Here's how the part is built. I have some questions about the finished solid (model axes, mm). A direction names the side the tool comes from. Coordinates: 2 decimals unless noted, no trailing zeros. Write each loop counter-clockwise with the first axis right and the second up, starting at its lowest first coordinate (ties: lowest second). Pieces come first, ordered by that corner, then holes.
```python
from build123d import *

# Parameters (mm, degrees)
F1_DEPTH = 903
F4_DEPTH = 5
F5_R     = 2


# Not quite as in the source:
# - a feature names something its author has since deleted; it is built from what else it names


with BuildPart() as f1:
    # F0 (on Right) → F1 (new body)
    with BuildSketch(Plane.YZ):
        Polygon((-295, 0), (0, 0), (0, 430), (-5, 430), (-5, 5), (-290, 5), (-290, 430), (-295, 430), align=None)
    extrude(amount=F1_DEPTH)

    # F3 (on offset) → F4 (join)
    with BuildSketch(Plane.YZ.offset(300)):
        Polygon((-230, 0), (-5, 0), (-5, 360), align=None)
    extrude(amount=F4_DEPTH)

    # F5
    f5_edges = [f1.edges().sort_by_distance(p)[0] for p in [
        (451.5, 0, 0),
        (451.5, -295, 0),
    ]]
    fillet(f5_edges, radius=F5_R)


solid = f1.part
```
1) Will these pins go through, and if not, where does the flat tip stop? pin 1 (5 mm diameter, centred on y = -156, z = 87.5, fed in from +X); pin 2 (6 mm diameter, centred on x = 108.5, y = -62.5, fed in from +Z).
Values follow:
pin 1: stops at x = 305
pin 2: stops at z = 5
2) Imagine slicing it at B-B on z = 327.5. Please give me the cut outline in (x, y).
Values follow:
outline: (0, -295) - (903, -295) - (903, -290) - (0, -290) - close; (0, -5) - (300, -5) - (300, -25.31) - (305, -25.31) - (305, -5) - (903, -5) - (903, 0) - (0, 0) - close
3) Imagine slicing it at A-A on y = -189. Please give me the cut outline in (x, z).
Values follow:
outline: (0, 0) - (903, 0) - (903, 5) - (305, 5) - (305, 65.6) - (300, 65.6) - (300, 5) - (0, 5) - close
4) On a 3-axis mill with a long thin cutter (end or side, diameter ignored), from which of +Z, -Z, +X, -X, +Y, -Y can I reach the whole of each face in a straight line? I mean faces 4 (the face through (302.465, -114.384, 184.985)), 5 (the face through (445, -295, 219)), 6 (the face through (445, -5, 220)), 7 (the face through (305, -68, 106)). Say none if no direction works.
Values follow:
face 4: +Z, +X, -X
face 5: +Z, -Z, +X, -X, -Y
face 6: +Z
face 7: +Z, +X
5) I need wall thicknesses on probe 1 along Y at (x, z) = (498, 99.5); probe 2 along Z at (x, y) = (800, -122.5); probe 3 along X at (y, z) = (-76.5, 118). Which ranges of each line are inside material? Lowest first, please.
Values follow:
probe 1: y = -295 to -290, -5 to 0
probe 2: z = 0 to 5
probe 3: x = 300 to 305
6) Imagine slicing it at C-C on x = 614. Please give me the cut outline in (y, z).
Values follow:
outline: (-295, 2) arc R2 ccw to (-293, 0) - (-2, 0) arc R2 ccw to (0, 2) - (0, 430) - (-5, 430) - (-5, 5) - (-290, 5) - (-290, 430) - (-295, 430) - close
7) Imagine slicing it at D-D on y = -104.5. Please give me the cut outline in (x, z), then the cut area to 3 significant figures.
Values follow:
outline: (0, 0) - (903, 0) - (903, 5) - (305, 5) - (305, 200.8) - (300, 200.8) - (300, 5) - (0, 5) - close
area: 5,490 mm2
8) We'd pull the mould along Y, two halves only. Please class faces 1 (the face through (300, -68, 106)), 2 (the face through (903, -290.2, 216)), 3 (the face through (445, 0, 213)): pulls with the +Y half, pulls with the -Y half, needs draft (parallel to the pull), parting line crosses it, or undercut.
Values follow:
face 1: undercut
face 2: needs draft
face 3: pulls with the +Y half
